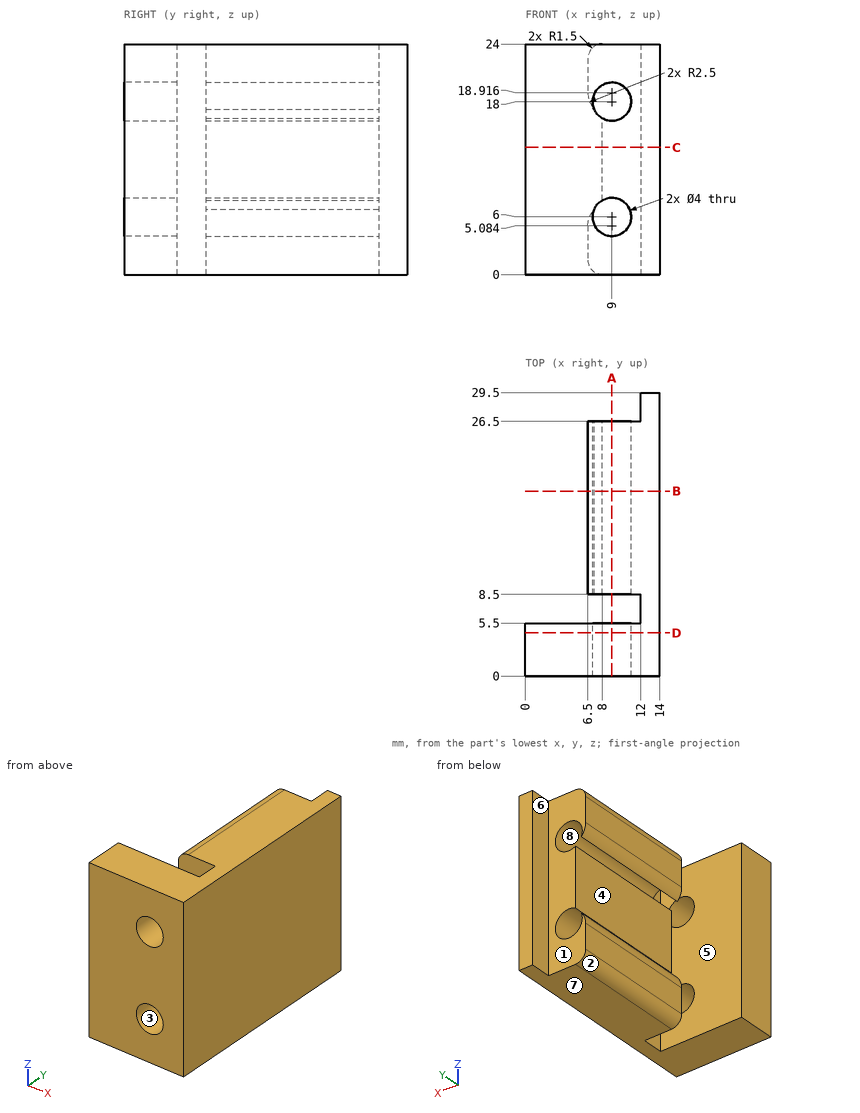
Job drawing, mm, ordinate dimensions from the low corner. One solid piece. A direction names the side the tool comes from. Give positions to 0.01 mm unless a question says otherwise; leave off trailing zeros. Loops run counter-clockwise (first coordinate to the right, second up) from the corner with the lowest first, then second, coordinate; pieces in that order, holes last. Notation, with made-up numbers: M -23,34.5 L -13,34.5 A4 ccw -13,41.5 Z; hole C -1,-37 d9. An arc over 180 degrees is marked long. Put each result on its own line as item: value. Start each with the question number.
1) Saw through at C-C (z = 13.25). List the corners of the cut face in (x, y), then the cut area to 3 significant figures.
2) Saw through at B-B (y = 19.25). List the corners of the cut face in (x, z).
3) 3-axis set-ups, long thin cutter, end or side, ignore diameter. For the marked faces 1, 2, 3, 4 and 5: which of +Z, -Z, +X, -X, +Y, -Y reach the whole face in a straight line?
4) Saw through at A-A (x = 9). List the corners of the cut face in (y, z).
5) Flat gauge pins, fed straight in: pin 1 (0.9 mm diameter, centred on y = 7, z = 17.5, fed in from -X); pin 2 (5 mm diameter, centred on x = 9, z = 6, fed in from +Y); pin 3 (1.8 mm diameter, centred on y = 21.5, z = 3.5, fed in from -X). Where does each tip first touch, or does it go through?
6) Probe probe 1 along Z at (x, y) = (9, 15.25); probe 2 along X at (y, z) = (3.05, 18); probe 3 along X at (y, z) = (14, 10.25). List the from-to ranges inside material, lowest first.
7) Pull direction Z, two halves, no side cores. Call the marked faces 6, 7 and 8: +Z half, -Z half, draft (parallel to the pull), parting line (faces both ways), or undercut.
8) Saw through at D-D (y = 4.5). List the corners of the cut face in (x, z), then the cut area to 3 significant figures.
Numbers:
1. outline: M 0,0 L 14,0 L 14,29.5 L 12,29.5 L 12,26.5 L 8,26.5 L 8,8.5 L 12,8.5 L 12,5.5 L 0,5.5 Z
1. area: 197 mm^2
2. outline: M 6.5,1.5 A1.5 ccw 8,0 L 14,0 L 14,24 L 8,24 A1.5 ccw 6.5,22.5 L 6.5,18.92 A2.5 ccw 7.15,17.23 A2 cw long 8,16.27 L 8,7.73 A2 cw long 7.15,6.77 A2.5 ccw 6.5,5.08 Z
3. face 1: +Z, -Z, -X, +Y
3. face 2: -Z, -X, +Y
3. face 3: +Y, -Y
3. face 4: -X, +Y
3. face 5: +Z, -Z, -X
4. outline: M 0,0 L 5.5,0 L 5.5,4 L 0,4 Z; M 0,8 L 5.5,8 L 5.5,16 L 0,16 Z; M 0,20 L 5.5,20 L 5.5,24 L 0,24 Z; M 8.5,0 L 26.5,0 L 26.5,4 L 8.5,4 Z; M 8.5,8 L 26.5,8 L 26.5,16 L 8.5,16 Z; M 8.5,20 L 26.5,20 L 26.5,24 L 8.5,24 Z
5. pin 1: x = 12
5. pin 2: y = 26.5
5. pin 3: x = 6.5
6. probe 1: 0 to 4, 8 to 16, 20 to 24
6. probe 2: 0 to 7, 11 to 14
6. probe 3: 8 to 14
7. face 6: draft
7. face 7: -Z half
7. face 8: undercut
8. outline: M 0,0 L 14,0 L 14,24 L 0,24 Z; hole C 9,6 d4; hole C 9,18 d4
8. area: 311 mm^2
